The model under review builds one solid part; all positions refer to its coordinate system, in mm. Face numbers are marked on the shaded views. A direction names the side the tool comes from. Round coordinates to 2 decimals unless told otherwise and drop trailing zeros. Order: outer loops, then holes, each group sorted by start corner. A loop starts at its lowest first (then second) coordinate and runs counter-clockwise, first axis right, second up. Notation, with made-up numbers: M 64,77 L 84,77 A33 cw 84,113 Z; hole C 16.25,27 d4. An arc over 180 degrees is marked long. Answer as a JSON object with one key per item and string values. Group by question number.
1. Add section A-A on x = 52. State the section outline as (y, z) points, and give its area (3 significant figures).
2. To check wall thickness, follow probe 1 along Y at (x, z) = (7, 27); probe 2 along X at (y, z) = (-6, 17); probe 3 along Z at (x, y) = (17.5, 23.5). State the ranges of each line that lie inside material, in increasing order. Write a range as [from, to].
3. Add section B-B on z = 36.5. State the section outline as (x, y) points.
4. Add section D-D on y = 12. State the section outline as (x, z) points.
5. Machinability: for the marked faces 1 and 2, which of the approach directions +Z, -Z, +X, -X, +Y, -Y give a long, thin tool a straight path to every point of the face, cutting with its end or side? Answer none if there is none.
6. Add section C-C on z = 11.5. State the section outline as (x, y) points.
7. Clearance check with flat-ended pins moving along their axes: P1, Ø5, axis at x = 35, y = 32.5, coming from the +Z side; P2, Ø0.9, axis at x = -62, y = -10.5, coming from the -Z side; P3, Ø0.9, axis at x = -61, y = 32, coming from the +Z side. State where each tip first meets the part, or that it passes through.
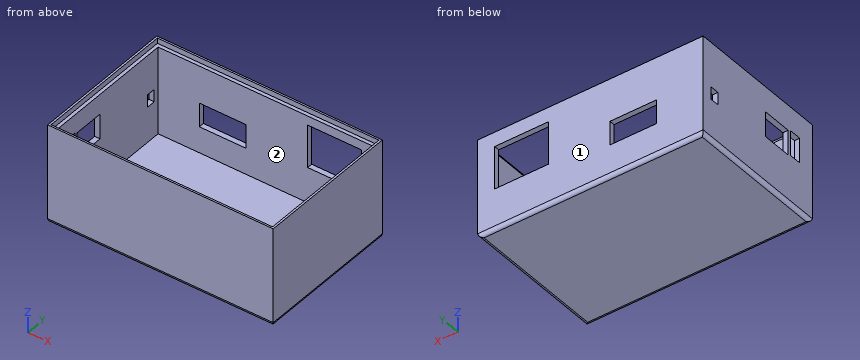
```python
from build123d import *

# Parameters (mm, degrees)
SKETCH_W        = 126
SKETCH_H        = 81
SKETCH_W_2      = 120
SKETCH_H_2      = 75
PAD_DEPTH       = 49
SKETCH001_W     = 126
SKETCH001_H     = 81
PAD001_DEPTH    = 3
SKETCH006_W     = 26.07241
SKETCH006_H     = 13.378264
POCKET002_DEPTH = 5
SKETCH007_W     = 126
SKETCH007_H     = 81
SKETCH007_W_2   = 123.756296
SKETCH007_H_2   = 79.00857
PAD004_DEPTH    = 3
SKETCH003_W     = 17
SKETCH003_H     = 14
SKETCH003_W_2   = 6.8
POCKET_DEPTH    = 5
SKETCH004_W     = 30
SKETCH004_H     = 24
POCKET003_DEPTH = 10
FILLET_R        = 2
SKETCH008_W     = 5
SKETCH008_H     = 7
POCKET004_DEPTH = 5


with BuildPart() as part:
    # Sketch → Pad (new body)
    with BuildSketch(Plane.XY):
        Rectangle(SKETCH_W, SKETCH_H)
        Rectangle(SKETCH_W_2, SKETCH_H_2, mode=Mode.SUBTRACT)
    extrude(amount=PAD_DEPTH)

    # Sketch001 (on Face9 of Pad) → Pad001 (join)
    with BuildSketch(Plane(origin=(0, 0, 0), x_dir=(1, 0, 0), z_dir=(0, 0, -1))):
        Rectangle(SKETCH001_W, SKETCH001_H)
    extrude(amount=PAD001_DEPTH)

    # Sketch006 → Pocket002 (cut)
    with BuildSketch(Plane(origin=(0, 40.5, 0), x_dir=(-1, 0, 0), z_dir=(0, 1, 0))):
        with Locations((23.94159, 21.396661)):
            Rectangle(SKETCH006_W, SKETCH006_H)
    extrude(amount=-POCKET002_DEPTH, mode=Mode.SUBTRACT)

    # Sketch007 (on Face4 of Pocket002) → Pad004 (join)
    with BuildSketch(Plane.XY.offset(49)):
        Rectangle(SKETCH007_W, SKETCH007_H)
        Rectangle(SKETCH007_W_2, SKETCH007_H_2, mode=Mode.SUBTRACT)
    extrude(amount=PAD004_DEPTH)

    # Sketch003 → Pocket (cut)
    with BuildSketch(Plane(origin=(-63, 0, 0), x_dir=(0, -1, 0), z_dir=(-1, 0, 0))):
        with Locations((14.1, 30.857126)):
            Rectangle(SKETCH003_W, SKETCH003_H)
        with Locations((27.8, 31.697018)):
            Rectangle(SKETCH003_W_2, SKETCH003_H)
    extrude(amount=-POCKET_DEPTH, mode=Mode.SUBTRACT)

    # Sketch004 → Pocket003 (cut)
    with BuildSketch(Plane(origin=(0, 47.5, 0), x_dir=(-1, 0, 0), z_dir=(0, 1, 0))):
        with Locations((-38.538937, 31.890343)):
            Rectangle(SKETCH004_W, SKETCH004_H)
    extrude(amount=-POCKET003_DEPTH, mode=Mode.SUBTRACT)

    # Fillet
    fillet_edges = [part.edges().sort_by_distance(p)[0] for p in [
        (0, -40.5, -3),
        (63, 0, -3),
        (0, 40.5, -3),
        (-63, 0, -3),
    ]]
    fillet(fillet_edges, radius=FILLET_R)

    # Sketch008 (on Face11 of Fillet) → Pocket004 (cut)
    with BuildSketch(Plane(origin=(-63, 0, 0), x_dir=(0, -1, 0), z_dir=(-1, 0, 0))):
        with Locations((-32.098774, 23.391483)):
            Rectangle(SKETCH008_W, SKETCH008_H)
    extrude(amount=-POCKET004_DEPTH, mode=Mode.SUBTRACT)


solid = part.part
```
Recorded:
{
 "1": {"outline": "M -40.5,-1 A2 ccw -38.5,-3 L 38.5,-3 A2 ccw 40.5,-1 L 40.5,19.89 L 37.5,19.89 L 37.5,0 L -37.5,0 L -37.5,49 L -39.5,49 L -39.5,52 L -40.5,52 Z; M 37.5,43.89 L 40.5,43.89 L 40.5,52 L 39.5,52 L 39.5,49 L 37.5,49 Z", "area": "469 mm²"},
 "2": {"probe 1": "y = [-40.5, -37.5], [37.5, 40.5]", "probe 2": "x = [-63, -60], [60, 63]", "probe 3": "z = [-3, 0]"},
 "3": {"outline": "M -63,-40.5 L 63,-40.5 L 63,40.5 L 53.54,40.5 L 53.54,37.5 L 60,37.5 L 60,-37.5 L -60,-37.5 L -60,-31.2 L -63,-31.2 Z; M -63,-24.4 L -60,-24.4 L -60,-22.6 L -63,-22.6 Z; M -63,-5.6 L -60,-5.6 L -60,37.5 L 23.54,37.5 L 23.54,40.5 L -63,40.5 Z"},
 "4": {"outline": "M -63,-1 A2 ccw -61,-3 L 61,-3 A2 ccw 63,-1 L 63,52 L 61.88,52 L 61.88,49 L 60,49 L 60,0 L -60,0 L -60,49 L -61.88,49 L -61.88,52 L -63,52 Z"},
 "5": {"face 1": "+Z, -Z, +X, -X, +Y", "face 2": "+Z"},
 "6": {"outline": "M -63,-40.5 L 63,-40.5 L 63,40.5 L -63,40.5 Z; hole M -60,-37.5 L 60,-37.5 L 60,37.5 L -60,37.5 Z"},
 "7": {"P1": "stops at z = 0", "P2": "stops at z = -2.92", "P3": "stops at z = 49"}
}
